Could you check a few things on this model? Use its own coordinates, in mm. Coordinates: 2 decimals unless noted, no trailing zeros. One line per item, written item: value. Start each with the question number.
(1) I'm going to push flat-ended pins straight in: P1, Ø1.4, axis at x = 39, z = 1.5, coming from the +Y side; P2, Ø3.5, axis at y = 15.5, z = 3.5, coming from the +X side; P3, Ø1.9, axis at x = 39.5, z = 2.5, coming from the -Y side. Where does each tip first touch, or does it pass through?
(2) If I drill on line 1 along Y through (x, z) = (19.05, 1.5); line 2 along Y through (x, z) = (38.1, 1.5); line 3 along X through (y, z) = (11.5, 4.5) (3 decimals), over which ranges is the centre line in solid material (lowest first)? Write a range as from..to.
(3) If we section it at A-A on z = 5.25: Count the separate pieces of the cut face and the enclosed holes in it, then the cut area to 3 significant figures.
```python
from build123d import *

# Parameters (mm, degrees)
SKETCH1_W                                   = 152.4
SKETCH1_H                                   = 215.9
BOSS_EXTRUDE1_DEPTH                         = 6.35
SKETCH2_R                                   = 1.524
CUT_EXTRUDE1_DEPTH                          = 265.346160366
SKETCH4_R                                   = 1.524
CUT_EXTRUDE2_DEPTH                          = 265.346160366
SKETCH5_R                                   = 1.524
CUT_EXTRUDE3_DEPTH                          = 265.346160366
SKETCH9_W                                   = 81.28
SKETCH9_H                                   = 6.35
CUT_EXTRUDE9_DEPTH                          = 265.346160366
CUT_EXTRUDE10_DEPTH                         = 265.346160366
SKETCH11_W                                  = 50.8
SKETCH11_H                                  = 203.2
CUT_EXTRUDE11_DEPTH                         = 61.976
SKETCH13_W                                  = 4.318
SKETCH13_H                                  = 4.439032047
SKETCH13_H_2                                = 4.376890529
CUT_EXTRUDE12_DEPTH                         = 6.35
SKETCH14_W                                  = 4.318
SKETCH14_H                                  = 4.368724603
CUT_EXTRUDE13_DEPTH                         = 6.35
SKETCH15_W                                  = 125.806146595
SKETCH15_H                                  = 228.6
GETTING_RID_OF_TOP_IMPINGES_WITH_DOOR_DEPTH = 265.346160366


with BuildPart() as part:
    # Sketch1 → Boss-Extrude1 (new body)
    with BuildSketch(Plane.XY):
        with Locations((76.2, 107.95)):
            Rectangle(SKETCH1_W, SKETCH1_H)
    extrude(amount=BOSS_EXTRUDE1_DEPTH)

    # Sketch2 → Cut-Extrude1 (cut, through all)
    with BuildSketch(Plane.XY.offset(6.35)):
        with Locations((19.05, 212.725)):
            Circle(SKETCH2_R)
        with Locations(Location((133.35, 212.725, 0), (0, 0, 180))):
            Circle(SKETCH2_R)
        with Locations((133.35, 3.175)):
            Circle(SKETCH2_R)
        with Locations(Location((19.05, 3.175, 0), (0, 0, 180))):
            Circle(SKETCH2_R)
    extrude(amount=-CUT_EXTRUDE1_DEPTH, mode=Mode.SUBTRACT)

    # Sketch4 → Cut-Extrude2 (cut, through all)
    with BuildSketch(Plane.XY.offset(6.35)):
        with Locations(Location((95.25, 133.35, 0), (0, 0, 180))):
            Circle(SKETCH4_R)
        with Locations((95.25, 82.55)):
            Circle(SKETCH4_R)
    extrude(amount=-CUT_EXTRUDE2_DEPTH, mode=Mode.SUBTRACT)

    # Sketch5 → Cut-Extrude3 (cut, through all)
    with BuildSketch(Plane.XY.offset(6.35)):
        with Locations((38.1, 133.35)):
            Circle(SKETCH5_R)
        with Locations(Location((38.1, 82.55, 0), (0, 0, 180))):
            Circle(SKETCH5_R)
    extrude(amount=-CUT_EXTRUDE3_DEPTH, mode=Mode.SUBTRACT)

    # Sketch9 → Cut-Extrude9 (cut, through all)
    with BuildSketch(Plane(origin=(0, 0, 0), x_dir=(-1, 0, 0), z_dir=(0, 0, -1))):
        with Locations((-76.2, 212.725)):
            Rectangle(SKETCH9_W, SKETCH9_H)
        with Locations((-76.2, 3.175)):
            Rectangle(SKETCH9_W, SKETCH9_H)
    extrude(amount=-CUT_EXTRUDE9_DEPTH, mode=Mode.SUBTRACT)

    # Sketch10 → Cut-Extrude10 (cut, through all)
    with BuildSketch(Plane(origin=(0, 0, 0), x_dir=(-1, 0, 0), z_dir=(0, 0, -1))):
        Polygon((-111.9632, 6.35), (-109.0168, 6.35), (-109.0168, 10.31875), (-107.315, 10.31875), (-107.315, 12.7), (-109.0168, 12.7), (-109.0168, 19.05), (-111.9632, 19.05), (-111.9632, 12.7), (-113.665, 12.7), (-113.665, 10.31875), (-111.9632, 10.31875), align=None)
        Polygon((-107.315, 205.58125), (-107.315, 203.2), (-109.0168, 203.2), (-109.0168, 196.85), (-111.9632, 196.85), (-111.9632, 203.2), (-113.665, 203.2), (-113.665, 205.58125), (-111.9632, 205.58125), (-111.9632, 209.55), (-109.0168, 209.55), (-109.0168, 205.58125), align=None)
        Polygon((-43.3832, 205.58125), (-45.085, 205.58125), (-45.085, 203.2), (-43.3832, 203.2), (-43.3832, 196.85), (-40.4368, 196.85), (-40.4368, 203.2), (-38.735, 203.2), (-38.735, 205.58125), (-40.4368, 205.58125), (-40.4368, 209.55), (-43.3832, 209.55), align=None)
        Polygon((-38.735, 10.31875), (-38.735, 12.7), (-40.4368, 12.7), (-40.4368, 19.05), (-43.3832, 19.05), (-43.3832, 12.7), (-45.085, 12.7), (-45.085, 10.31875), (-43.3832, 10.31875), (-43.3832, 6.35), (-40.4368, 6.35), (-40.4368, 10.31875), align=None)
    extrude(amount=-CUT_EXTRUDE10_DEPTH, mode=Mode.SUBTRACT)

    # Sketch11 → Cut-Extrude11 (cut)
    with BuildSketch(Plane(origin=(0, 0, 0), x_dir=(-1, 0, 0), z_dir=(0, 0, -1))):
        with Locations((-76.2, 107.95)):
            Rectangle(SKETCH11_W, SKETCH11_H)
    extrude(amount=-CUT_EXTRUDE11_DEPTH, mode=Mode.SUBTRACT)


with BuildPart() as cut_extrude11_piece_1:
    # of the separate pieces the step leaves, piece 1, a body of its own (cut_extrude11_pieces)
    add(part.part.solids().sort_by_distance((101.6, 209.55, 0))[0])

    # Sketch15 → Getting rid of top, impinges with door (cut, through all)
    with BuildSketch(Plane.XY.offset(6.35)):
        with Locations((143.333722475, 114.3)):
            Rectangle(SKETCH15_W, SKETCH15_H)
    extrude(amount=-GETTING_RID_OF_TOP_IMPINGES_WITH_DOOR_DEPTH, mode=Mode.SUBTRACT)


with BuildPart() as cut_extrude11_piece_2:
    # of the separate pieces the step leaves, piece 2, a body of its own (cut_extrude11_pieces)
    add(part.part.solids().sort_by_distance((0, 0, 0))[0])

    # Sketch13 → Cut-Extrude12 (cut)
    with BuildSketch(Plane(origin=(0, 0, 0), x_dir=(-1, 0, 0), z_dir=(0, 0, -1))):
        with Locations((-48.641, 15.139283389)):
            Rectangle(SKETCH13_W, SKETCH13_H)
        with Locations((-48.641, 202.163626755)):
            Rectangle(SKETCH13_W, SKETCH13_H_2)
    extrude(amount=-CUT_EXTRUDE12_DEPTH, mode=Mode.SUBTRACT)

    # Sketch14 → Cut-Extrude13 (cut)
    with BuildSketch(Plane(origin=(0, 0, 0), x_dir=(-1, 0, 0), z_dir=(0, 0, -1))):
        with Locations((-48.641, 108.744312397)):
            Rectangle(SKETCH14_W, SKETCH14_H)
    extrude(amount=-CUT_EXTRUDE13_DEPTH, mode=Mode.SUBTRACT)


solid = cut_extrude11_piece_2.part
```
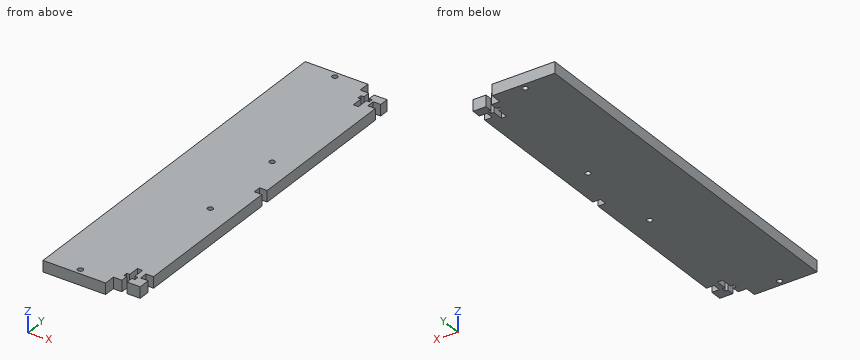
Values:
1. P1: stops at y = 209.55
1. P2: stops at x = 46.48
1. P3: stops at y = 6.35
2. line 1: y = 0..1.65, 4.7..211.2, 214.25..215.9
2. line 2: y = 6.35..81.03, 84.07..131.83, 134.87..209.55
2. line 3: x = 0..38.735, 45.085..50.8
3. separate pieces: 1
3. enclosed holes: 4
3. area: 10,600 mm2
